For this review, take the finished solid that the model builds, in its own axes (mm). A direction names the side the tool comes from. Coordinates: 2 decimals unless noted, no trailing zeros. Write each loop counter-clockwise with the first axis right and the second up, starting at its lowest first coordinate (ties: lowest second). Pieces come first, ordered by that corner, then holes.
1) We need section D-D on z = 2.5. Write out the cut boundary in (x, y).
2) For faces 4 (the face through (0, 7, -3.65)), 5 (the face through (-6, 4, 3.65)), 6 (the face through (-2.33, -1.71, 0.38)), 7 (the face through (9, -2, 0)), 8 (the face through (1, 7, 3.65)), list the 3-axis set-ups (+Z, -Z, +X, -X, +Y, -Y) from which the entire face can be reached by the end or side of a thin tool; tool diameter is ignored.
3) To check wall thickness, follow line 1 along Y through (x, z) = (0, -5.75); line 2 along Y through (x, z) = (-5, 7.5); line 3 along X through (y, z) = (2.75, 0). State the ranges of each line that lie inside material, in increasing order.
4) We need section C-C on x = 6.5. Write out the cut boundary in (y, z).
5) Mouldability with a two-part tool opening along X and no side actions: class faces 1 (the face through (-2, 8.825, 2)), 2 (the face through (4, 3, -1)), 3 (the face through (0.47, -2.1, -5.39)) as pulls with the +X half, pulls with the -X half, needs draft (parallel to the pull), parting line crosses it, or undercut.
6) We need section A-A on x = -2.75. Write out the cut boundary in (y, z), then the cut area to 3 significant figures.
7) Insertion check: P1, Ø8, axis at x = 0.5, z = 10.5, coming from the +Y side; P2, Ø3, axis at y = 5, z = 2, coming from the +X side; P3, Ø5.5, axis at y = 0, z = 0, coming from the -X side. Each pin has a flat end and moves straight along its axis. Give the tip position at first contact, or say it passes through.
from build123d import *

# Parameters (mm, degrees)
SKETCH1_R               = 1.75
BOSS_EXTRUDE1_DEPTH     = 4
SKETCH2_R               = 2.15
CUT_EXTRUDE1_DEPTH      = 5
BOSS_EXTRUDE5_START     = -1.8499999
BOSS_EXTRUDE5_OUTLINE_R = 2
BOSS_EXTRUDE5_DEPTH     = 11.8499999
BOSS_EXTRUDE5_START_2   = -3
BOSS_EXTRUDE5_2_DEPTH   = 7.824935333
SKETCH3_R               = 2.15
CUT_EXTRUDE2_DEPTH      = 5
BOSS_EXTRUDE2_START     = 4
SKETCH4_W               = 8
SKETCH4_H               = 7.3
SKETCH4_R               = 2.15
BOSS_EXTRUDE2_DEPTH     = 4
BOSS_EXTRUDE3_START     = 4
SKETCH5_W               = 8
SKETCH5_H               = 7.3
SKETCH5_R               = 2.15
BOSS_EXTRUDE3_DEPTH     = 4
SKETCH6_R               = 0.4895
BOSS_EXTRUDE4_DEPTH     = 10
FILLET1_R               = 2


with BuildPart() as part:
    # Sketch1 → Boss-Extrude1 (new, symmetric)
    with BuildSketch(Plane(origin=(0, 0, 0), x_dir=(0, 0, -1), z_dir=(1, 0, 0))):
        with BuildLine():
            Line((-3.65, 4.824935233), (3.65, 4.824935233))
            ThreePointArc((3.65, 4.824935233), (4.277996026, 4.277996026), (4.824935233, 3.65))
            Line((4.824935233, 3.65), (4.824935233, -3.65))
            ThreePointArc((4.824935233, -3.65), (-4.277996026, -4.277996026), (-3.65, 4.824935233))
        make_face()
        Circle(SKETCH1_R, mode=Mode.SUBTRACT)
    extrude(amount=BOSS_EXTRUDE1_DEPTH, both=True)

    # Sketch2 → Cut-Extrude1 (cut)
    with BuildSketch(Plane(origin=(0, 4.824935233, 0), x_dir=(1, 0, 0), z_dir=(0, 1, 0))):
        with Locations(Location((0, 0, 0), (0, 0, 270))):
            Circle(SKETCH2_R)
    extrude(amount=-CUT_EXTRUDE1_DEPTH, mode=Mode.SUBTRACT)

    # Boss-Extrude5: read off the stored shape, not the designer's step
    # Boss-Extrude5 outline → Boss-Extrude5 (add)
    with BuildSketch(Plane(origin=(4, 0, 0), x_dir=(0, 0, -1), z_dir=(1, 0, 0)).offset(BOSS_EXTRUDE5_START)):
        Circle(BOSS_EXTRUDE5_OUTLINE_R)
    extrude(amount=BOSS_EXTRUDE5_DEPTH)

    # Boss-Extrude5 2 outline → Boss-Extrude5 2 (add)
    with BuildSketch(Plane(origin=(0, 0, 0), x_dir=(1, 0, 0), z_dir=(0, 1, 0)).offset(BOSS_EXTRUDE5_START_2)):
        with BuildLine():
            Line((2.1500001, -3), (2.15, 0))
            ThreePointArc((2.15, 0), (1.52027958, -1.52027958), (0, -2.15))
            Line((0, -2.15), (0, -3))
            Line((0, -3), (2.1500001, -3))
        make_face()
        with BuildLine():
            ThreePointArc((0, 2.15), (1.52027958, 1.52027958), (2.15, 0))
            Line((2.15, 0), (2.1500001, 3))
            Line((2.1500001, 3), (0, 3))
            Line((0, 3), (0, 2.15))
        make_face()
    extrude(amount=BOSS_EXTRUDE5_2_DEPTH)

    # Sketch3 → Cut-Extrude2 (cut)
    with BuildSketch(Plane(origin=(0, 0, -4.824935233), x_dir=(-1, 0, 0), z_dir=(0, 0, -1))):
        Circle(SKETCH3_R)
    extrude(amount=-CUT_EXTRUDE2_DEPTH, mode=Mode.SUBTRACT)

    # Sketch4 → Boss-Extrude2 (add)
    with BuildSketch(Plane(origin=(0, 4.824935233, 0), x_dir=(1, 0, 0), z_dir=(0, 1, 0)).offset(BOSS_EXTRUDE2_START)):
        Rectangle(SKETCH4_W, SKETCH4_H)
        with Locations(Location((0, 0, 0), (0, 0, 270))):
            Circle(SKETCH4_R, mode=Mode.SUBTRACT)
    extrude(amount=-BOSS_EXTRUDE2_DEPTH)

    # Sketch5 → Boss-Extrude3 (add)
    with BuildSketch(Plane(origin=(0, 0, -4.824935233), x_dir=(-1, 0, 0), z_dir=(0, 0, -1)).offset(BOSS_EXTRUDE3_START)):
        Rectangle(SKETCH5_W, SKETCH5_H)
        Circle(SKETCH5_R, mode=Mode.SUBTRACT)
    extrude(amount=-BOSS_EXTRUDE3_DEPTH)

    # Sketch6 → Boss-Extrude4 (add)
    with BuildSketch(Plane.XY.offset(3.65)):
        with BuildLine():
            Line((-2, 5.5445), (-5, 5.5445))
            ThreePointArc((-5, 5.5445), (-6.9895, 3.555), (-5, 1.5655))
            Line((-5, 1.5655), (-2, 1.5655))
            ThreePointArc((-2, 1.5655), (-0.0105, 3.555), (-2, 5.5445))
        make_face()
        with Locations((-5, 3.555)):
            Circle(SKETCH6_R, mode=Mode.SUBTRACT)
    extrude(amount=BOSS_EXTRUDE4_DEPTH)

    # Fillet1
    # the kernel refuses this fillet: 2 mm, written as the material it adds along each edge
    with BuildSketch(Plane(origin=(-2, 3.555, 3.65), x_dir=(-0.2477928617675286, -0.9688130354495952, 0), z_dir=(-0.9688130354495952, 0.2477928617675286, 0))) as fillet1_piece_1:
        with BuildLine():
            CenterArc((1.9895 + FILLET1_R, FILLET1_R), FILLET1_R, 180, 90)
            Line((1.9895 + FILLET1_R, 0), (1.9895, 0))
            Line((1.9895, 0), (1.9895, FILLET1_R))
        make_face()
    revolve(axis=Axis((-2, 3.555, 3.65), (0, 0, 1)), revolution_arc=194.346943464)
    with BuildSketch(Plane(origin=(-2, 5.5445, 3.65), x_dir=(0, 0, 1), z_dir=(-1, 0, 0))) as fillet1_piece_2:
        with BuildLine():
            CenterArc((FILLET1_R, FILLET1_R), FILLET1_R, 180, 90)
            Line((0, FILLET1_R), (0, 0))
            Line((0, 0), (FILLET1_R, 0))
        make_face()
    extrude(amount=2)


solid = part.part
Result:
1. outline: (-4, -5.51) - (4, -5.51) - (4, 8.82) - (-4, 8.82) - close
2. face 4: -Z, +X, -X, +Y
2. face 5: -Z, -X, +Y, -Y
2. face 6: -X
2. face 7: +X
2. face 8: +Z, +X, +Y
3. line 1: y = -3.65 to -2.15, 2.15 to 3.65
3. line 2: y = 1.57 to 3.07, 4.04 to 5.54
3. line 3: x = -4 to -2.15, 2.15 to 4
4. outline: circle Ø4 at (0, 0)
5. face 1: needs draft
5. face 2: pulls with the +X half
5. face 3: undercut
6. outline: (-3.65, -8.82) - (3.65, -8.82) - (3.65, -4.82) arc R6.05 ccw to (4.82, -3.65) - (8.82, -3.65) - (8.82, 3.65) - (7.54, 3.65) arc R2 cw to (5.54, 5.65) - (5.54, 13.65) - (1.57, 13.65) - (1.57, 5.84) arc R6.05 ccw to (-3.65, -4.82) - close; hole circle Ø3.5 at (0, 0)
6. area: 188 mm2
7. P1: stops at y = 5.54
7. P2: stops at x = 4
7. P3: stops at x = -4
